Autodesk Inventor part; units mm, degrees
ref_plane "MidSidePlane" through (0, 12, 0) normal (0, 1, 0) x (-1, 0, 0)
ref_plane "YZ Plane" through (0, 0, 0) normal (1, 0, 0) x (0, 1, 0)
ref_plane "XY Plane" through (0, 0, 0) normal (0, 0, 1) x (1, 0, 0)
sketch "Mount" plane through (0, 0, 0) normal (0, 0, 1) x (1, 0, 0)
  circle A0 centre (0, 0) radius 7.45
  dimension "d0" = 14.9
extrude "MountFeature" add sketch "Mount" along normal blind 10
sketch "Base" plane through (0, 0, 10) normal (0, 0, 1) x (1, 0, 0)
  circle A0 centre (0, 0) radius 7.45 construction
  circle A1 centre (0, 0) radius 9
  dimension "d3" = 18
extrude "BaseFeature" add sketch "Base" along normal blind 4
sketch "RodEndHole" plane through (0, 0, 14) normal (0, 0, 1) x (1, 0, 0)
  circle A0 centre (0, 0) radius 9
hole "RodEndHoleFeature" at (0, 0, 14) direction (0, 0, -1) diameter 4.917 end through all
chamfer "BaseChamferFeature" distance 1 angle 45 1 edges at (-9, 0, 14)
ref_plane "MidSidePlane" through (0, 12, 0) normal (0, 1, 0) x (-1, 0, 0)
sketch "MountHole" plane through (0, 12, 0) normal (0, 1, 0) x (-1, 0, 0)
  line L0 (-9, 10) -> (9, 10) construction
  line L1 (7.45, 0) -> (7.45, 10) construction
  line L2 (7.45, 10) -> (-7.45, 10) construction
  line L3 (-7.45, 0) -> (7.45, 0) construction
  point P0 (0, 5.5)
  dimension "d18" = 4.5
  dimension "d26" = 18
  dimension "d27" = 9
hole "MountHoleFeature" at (0, 12, 5.5) direction (0, -1, 0) diameter 2.459 end through all
properties part number "BackPair1PistonBottomCap"
For this review, take the finished solid that the model builds, in its own axes (mm). Round coordinates to 2 decimals unless told otherwise and drop trailing zeros. Write each loop counter-clockwise with the first axis right and the second up, starting at its lowest first coordinate (ties: lowest second). Pieces come first, ordered by that corner, then holes. Notation, with made-up numbers: (41, 23) -> (67, 23) arc R24 cw to (67, 52) -> close; hole circle Ø9 at (87, 27.5). An arc over 180 degrees is marked (long way). Use one line per item in the form item = value.
Q1. Consider section C-C (z = 5.5). State the section outline as (x, y) points, then the cut area to 3 significant figures.
Resolved:
outline = (-1.23, -7.35) -> (-1.23, -2.13) arc R2.46 cw to (-1.23, 2.13) -> (-1.23, 7.35) arc R7.45 ccw to start; (1.23, -7.35) arc R7.45 ccw to (1.23, 7.35) -> (1.23, 2.13) arc R2.46 cw to (1.23, -2.13) -> close
area = 130 mm²
Q2. Consider section D-D (z = 3). State the section outline as (x, y) points.
Resolved:
outline = circle Ø14.9 at (0, 0); hole circle Ø4.92 at (0, 0)
Q3. Clearance check with flat-ended pins moving along their axes: pin 1 Ø3 at (x, z) = (0, 5.5) entering from -Y; pin 2 Ø1 at (x, z) = (-7, 3) entering from +Y; pin 3 Ø8 at (x, z) = (-4.5, 10.5) entering from -Y. State where each tip first meets the part, or that it passes through.
Resolved:
pin_1 = -7.45
pin_2 = 3.64
pin_3 = -8.99
Q4. The part is to be moulded in two halves that separate along X. For faces 1 (the cylindrical face through (-0.108, 2.456, 6.902)), 2 (the flat face through (-3, 7, 10)), 3 (the cylindrical face through (-0.05, 4.75, 4.27)), 4 (the cylindrical face through (3.44, 6.61, 4.93)), say which applies: released by +X, released by -X, zero draft, split by the parting line, or undercut.
Resolved:
face_1 = undercut
face_2 = zero draft
face_3 = undercut
face_4 = split by the parting line
Q5. Consider section B-B (y = 0). State the section outline as (x, z) points.
Resolved:
outline = (-9, 10) -> (-7.45, 10) -> (-7.45, 0) -> (-2.46, 0) -> (-2.46, 14) -> (-8, 14) -> (-9, 13) -> close; (2.46, 0) -> (7.45, 0) -> (7.45, 10) -> (9, 10) -> (9, 13) -> (8, 14) -> (2.46, 14) -> close
Q6. Consider section A-A (x = 0). State the section outline as (y, z) points.
Resolved:
outline = (-9, 10) -> (-7.45, 10) -> (-7.45, 6.73) -> (-2.46, 6.73) -> (-2.46, 14) -> (-8, 14) -> (-9, 13) -> close; (-7.45, 0) -> (-2.46, 0) -> (-2.46, 4.27) -> (-7.45, 4.27) -> close; (2.46, 0) -> (7.45, 0) -> (7.45, 4.27) -> (2.46, 4.27) -> close; (2.46, 6.73) -> (7.45, 6.73) -> (7.45, 10) -> (9, 10) -> (9, 13) -> (8, 14) -> (2.46, 14) -> close
Q7. To check wall thickness, follow probe 1 along Y at (x, z) = (0, 10.25); probe 2 along Y at (x, z) = (0, 7.5); probe 3 along Z at (x, y) = (0, -4.05). State the ranges of each line that lie inside material, in increasing order. Write a range as from..to.
Resolved:
probe_1 = -9..-2.46, 2.46..9
probe_2 = -7.45..-2.46, 2.46..7.45
probe_3 = 0..4.27, 6.73..14
